Read the model definition and answer for the solid it produces. Units are mm, in the model's axes. A direction names the side the tool comes from. Give positions to 0.01 mm unless a question says otherwise; leave off trailing zeros. Loops run counter-clockwise (first coordinate to the right, second up) from the corner with the lowest first, then second, coordinate; pieces in that order, holes last. Notation, with made-up numbers: (56, 16.25) - (66, 16.25) arc R35 cw to (66, 51.25) - close; hole circle Ø6 at (60, 80). An arc over 180 degrees is marked (long way). Write item = value, one per line.
```python
from build123d import *

# Parameters (mm, degrees)
SKETCH1_W                = 50
SKETCH1_H                = 50
BOSS_EXTRUDE1_DEPTH      = 50
CUT_EXTRUDE1_DEPTH       = 87.602540378
CHAMFER1_SIZE            = 1.5
BOSS_EXTRUDE2_DEPTH      = 7
BOSS_EXTRUDE2_DEPTH_BACK = 10
SKETCH5_W                = 1
SKETCH5_H                = 7
SKETCH6_W                = 1.8
SKETCH6_H                = 1.8
CUT_EXTRUDE2_DEPTH       = 7


with BuildPart() as part:
    # Sketch1 → Boss-Extrude1 (new body)
    with BuildSketch(Plane.XY):
        with Locations((25, 25)):
            Rectangle(SKETCH1_W, SKETCH1_H)
    extrude(amount=BOSS_EXTRUDE1_DEPTH)

    # Sketch2 → Cut-Extrude1 (cut, through all)
    with BuildSketch(Plane.XZ):
        Polygon((36, 45.443650814), (36, 54.556349186), (29.556349186, 61), (20.443650814, 61), (14, 54.556349186), (14, 45.443650814), (20.443650814, 39), (29.556349186, 39), align=None)
    extrude(amount=-CUT_EXTRUDE1_DEPTH, mode=Mode.SUBTRACT)

    # Cut-Sweep1: sweep along a path in Sketch4
    with BuildLine(Plane(origin=(25, 0, 0), x_dir=(0, 0, -1), z_dir=(1, 0, 0))) as cut_sweep1_path:
        Line((-13.5, 0), (-13.5, 3))
        ThreePointArc((-13.5, 3), (-19.943650814, 18.556349186), (-35.5, 25))
        Line((-35.5, 25), (-50, 25))
    # Sketch3 → Cut-Sweep1 (sweep, cut)
    with BuildSketch(Plane.XZ):
        Polygon((29.556349186, 24.5), (20.443650814, 24.5), (14, 18.056349186), (14, 8.943650814), (20.443650814, 2.5), (29.556349186, 2.5), (36, 8.943650814), (36, 18.056349186), align=None)
    sweep(path=cut_sweep1_path.line, mode=Mode.SUBTRACT)

    # Chamfer1
    chamfer1_edges = [part.edges().sort_by_distance(p)[0] for p in [
        (50, 25, 50),
        (43, 0, 50),
        (7, 50, 50),
        (36, 25, 50),
        (14, 25, 50),
        (14, 50, 47.721825407),
        (36, 50, 47.721825407),
        (36, 0, 47.721825407),
        (43, 50, 50),
        (14, 0, 47.721825407),
        (17.221825407, 0, 42.221825407),
        (32.778174593, 0, 42.221825407),
        (32.778174593, 50, 42.221825407),
        (17.221825407, 50, 42.221825407),
        (0, 25, 50),
        (25, 50, 0),
        (50, 25, 0),
        (25, 0, 0),
        (0, 25, 0),
        (7, 0, 50),
        (0, 50, 25),
        (50, 50, 25),
        (50, 0, 25),
        (0, 0, 25),
    ]]
    chamfer(chamfer1_edges, length=CHAMFER1_SIZE)

    # Sketch5 → Boss-Extrude2 (add, two sides: drawn at the far end of the back side and taken through both)
    with BuildSketch(Plane.XY.offset(50).offset(-BOSS_EXTRUDE2_DEPTH_BACK)):
        with Locations((0.5, 25)):
            Rectangle(SKETCH5_W, SKETCH5_H)
    extrude(amount=BOSS_EXTRUDE2_DEPTH + BOSS_EXTRUDE2_DEPTH_BACK)

    # Sketch6 → Cut-Extrude2 (cut)
    with BuildSketch(Plane(origin=(1, 0, 0), x_dir=(0, 0, -1), z_dir=(1, 0, 0))):
        with Locations((-53.6, 25)):
            Rectangle(SKETCH6_W, SKETCH6_H)
    extrude(amount=-CUT_EXTRUDE2_DEPTH, mode=Mode.SUBTRACT)


solid = part.part
```
1) A cutting plane is placed at A-A on x = 21.5. Determine the outline of the cut face in (y, z), then the cut area to 3 significant figures.
Output:
outline = (0, 1.5) - (1.5, 0) - (48.5, 0) - (50, 1.5) - (50, 39) - (36, 39) - (36, 35.5) arc R33 cw to (3, 2.5) - (0, 2.5) - close; (0, 24.5) - (3, 24.5) arc R11 ccw to (14, 35.5) - (14, 39) - (0, 39) - close
area = 1,040 mm²
2) A cutting plane is placed at B-B on y = 42. Determine the outline of the cut face in (x, z).
Output:
outline = (0, 1.5) - (1.5, 0) - (48.5, 0) - (50, 1.5) - (50, 48.5) - (48.5, 50) - (37.5, 50) - (36, 48.5) - (36, 45.44) - (29.56, 39) - (20.44, 39) - (14, 45.44) - (14, 48.5) - (12.5, 50) - (1.5, 50) - (0, 48.5) - close
3) A tool of negligible diameter and unlimited length cuts with its end or side. For faces 5 (the face through (33.57, 49.24, 41.97)), 6 (the face through (17.177, 8.734, 42.267)), 7 (the face through (34.255, 22.791, 15.269)), 8 (the face through (25, 2, 24.5)), 9 (the face through (13.3, 0.8, 46.7)), from which of +Z, -Z, +X, -X, +Y, -Y can it reach the whole face along a straight path? Write none if from no direction.
Output:
face_5 = +Z, +Y
face_6 = +Z, +Y, -Y
face_7 = none
face_8 = -Y
face_9 = +Z, -Y
4) Find the intervals of material crossed by probe 1 along X at (y, z) = (10.5, 14); probe 2 along Y at (x, z) = (16, 27); probe 3 along Z at (x, y) = (24.5, 40), in increasing order.
Output:
probe_1 = 0 to 14, 36 to 50
probe_2 = 0 to 15.89, 30.26 to 50
probe_3 = 0 to 39
5) The mould has two halves that part along X. Classify faces 1 (the face through (50, 25, 25)), 2 (the face through (6.9, 49.2, 49.3)), 3 (the face through (32.733, 1.521, 5.677)), 4 (the face through (36.7, 0.8, 46.6)): pulls with the +X half, pulls with the -X half, needs draft (parallel to the pull), parting line crosses it, or undercut.
Output:
face_1 = pulls with the +X half
face_2 = needs draft
face_3 = undercut
face_4 = undercut
6) A cutting plane is placed at D-D on x = 40.5. Determine the outline of the cut face in (y, z), then the cut area to 3 significant figures.
Output:
outline = (0, 1.5) - (1.5, 0) - (48.5, 0) - (50, 1.5) - (50, 48.5) - (48.5, 50) - (1.5, 50) - (0, 48.5) - close
area = 2,500 mm²
7) A cutting plane is placed at C-C on z = 40.5. Determine the outline of the cut face in (x, y), then the cut area to 3 significant figures.
Output:
outline = (0, 1.5) - (1.5, 0) - (16.82, 0) - (18.94, 1.5) - (18.94, 15.5) - (14, 20.44) - (14, 29.56) - (18.94, 34.5) - (18.94, 48.5) - (16.82, 50) - (1.5, 50) - (0, 48.5) - close; (31.06, 1.5) - (33.18, 0) - (48.5, 0) - (50, 1.5) - (50, 48.5) - (48.5, 50) - (33.18, 50) - (31.06, 48.5) - (31.06, 34.5) - (36, 29.56) - (36, 20.44) - (31.06, 15.5) - close
area = 1,740 mm²
8) Each of these flat-tipped pins is pushed along its axis until it touches: P1, Ø4, axis at x = 22, y = 10, coming from the +Z side; P2, Ø12, axis at x = 39.5, y = 8, coming from the +Z side; P3, Ø0.8, axis at x = 0.5, z = 54, coming from the +Y side. Where does it stop, or does it pass through?
Output:
P1 = 39.44
P2 = 50
P3 = 28.5
